Source: three-view drawing plus pictorial views. Frame: mm from the lowest corner of the part. Round coordinates to 2 decimals unless told otherwise and drop trailing zeros. Write each loop counter-clockwise with the first axis right and the second up, starting at its lowest first coordinate (ties: lowest second). Pieces come first, ordered by that corner, then holes. Notation, with made-up numbers: M -23.75,59 L 29.25,59 A23 ccw 29.25,76 Z; hole C 33.5,84 d1. An arc over 180 degrees is marked long. Put each result on its own line as item: value. Start each with the question number.
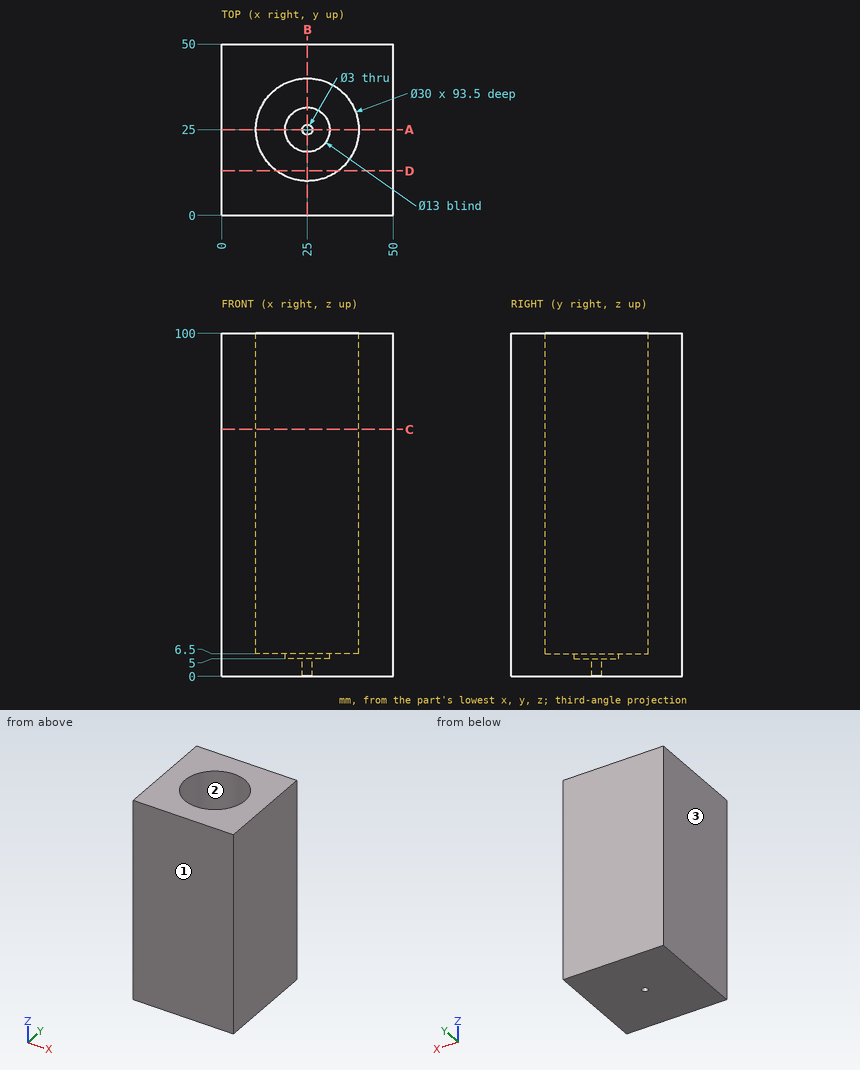
(1) Contact query for flat-ended pins moving along their axis: P1, Ø6, axis at x = 19.5, y = 28, coming from the +Z side; P2, Ø2.5, axis at x = 25, y = 25, coming from the +Z side. Output: stop coordinate, or through.
(2) Section query A-A (y = 25). Return loops of the section in (x, z), and give its area (3 significant figures).
(3) Section query D-D (y = 13). Return loops of the section in (x, z), and give its area (3 significant figures).
(4) Ray query, line 1 along Y through (x, z) = (25, 3.25); line 2 along Y through (x, z) = (25, 67.5). Return the intervals inside material, ascending.
(5) Pull-direction query (Y, two-part tool) for the marked faces 1, 2 and 3; classes: +Y half, -Y half, draft (parallel to the pull), parting line (faces both ways), or undercut.
(6) Section query C-C (z = 72). Return loops of the section in (x, y).
Entries:
1. P1: z = 6.5
1. P2: through
2. outline: M 0,0 L 23.5,0 L 23.5,5 L 18.5,5 L 18.5,6.5 L 10,6.5 L 10,100 L 0,100 Z; M 26.5,0 L 50,0 L 50,100 L 40,100 L 40,6.5 L 31.5,6.5 L 31.5,5 L 26.5,5 Z
2. area: 2,160 mm2
3. outline: M 0,0 L 50,0 L 50,100 L 34,100 L 34,6.5 L 16,6.5 L 16,100 L 0,100 Z
3. area: 3,320 mm2
4. line 1: 0 to 23.5, 26.5 to 50
4. line 2: 0 to 10, 40 to 50
5. face 1: -Y half
5. face 2: undercut
5. face 3: draft
6. outline: M 0,0 L 50,0 L 50,50 L 0,50 Z; hole C 25,25 d30
